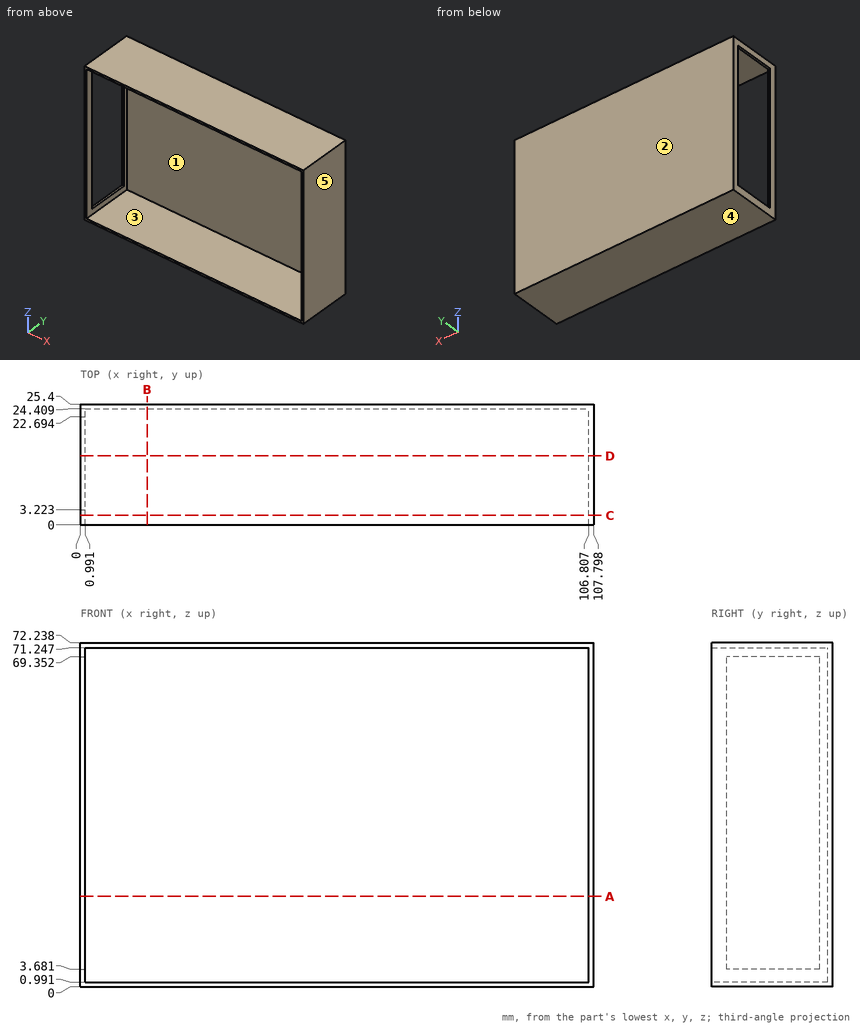
Study the drawing (mm; zero at the part's minimum x, y, z) and answer. A direction names the side the tool comes from. Coordinates: 2 decimals unless noted, no trailing zeros. Loops run counter-clockwise (first coordinate to the right, second up) from the corner with the lowest first, then second, coordinate; pieces in that order, holes last. Notation, with made-up numbers: M 55.5,89 L 63.5,89 A18 ccw 63.5,93 Z; hole C 39.25,75.5 d1. An arc over 180 degrees is marked long. Answer in a Markdown table with one row per item. Add a question column.
1. A tool of negligible diameter and unlimited length cuts with its end or side. For the marked faces 1 and 2, from which of +Z, -Z, +X, -X, +Y, -Y can it reach the whole face along a straight path? Write none if from no direction.
2. The mould has two halves that part along X. Classify the marked faces 3, 4 and 5: pulls with the +X half, pulls with the -X half, needs draft (parallel to the pull), parting line crosses it, or undercut.
3. Find section C-C, the plane y = 2. Write down the section's boundary in (x, z).
4. Find section D-D, the plane y = 14.5. Write down the section's boundary in (x, z).
5. Find section B-B, the plane x = 14. Write down the section's boundary in (y, z), then the cut area to 3 significant figures.
6. Find section A-A, the plane z = 19. Write down the section's boundary in (x, y) (1 decimal), then the cut area to 3 significant figures.
7. Consider L1, parallel to Z at x = 11.5, y = 14.75; L2, parallel to Y at x = 98, z = 60.5; L3, parallel to X at y = 12.25, z = 22. Determine where each line is inside the solid, lowest interval first.
8. Flat-ended cylindrical pins translate along their axes: P1, Ø0.8, axis at x = 0.5, y = 16.5, coming from the -Z side; P2, Ø21, axis at x = 50, z = 34, coming from the -Y side. Find the tip coordinate at first contact, or state that the pin passes through.
Reported:
| question | item | result |
|---|---|---|
| 1 | face 1 | -Y |
| 1 | face 2 | +Z, -Z, +X, -X, +Y |
| 2 | face 3 | undercut |
| 2 | face 4 | needs draft |
| 2 | face 5 | pulls with the +X half |
| 3 | outline | M 0,0 L 107.8,0 L 107.8,72.24 L 0,72.24 Z; hole M 0.99,0.99 L 106.81,0.99 L 106.81,71.25 L 0.99,71.25 Z |
| 4 | outline | M 0,0 L 107.8,0 L 107.8,72.24 L 0,72.24 L 0,69.35 L 0.99,69.35 L 0.99,71.25 L 106.81,71.25 L 106.81,0.99 L 0.99,0.99 L 0.99,3.68 L 0,3.68 Z |
| 5 | outline | M 0,0 L 25.4,0 L 25.4,72.24 L 0,72.24 L 0,71.25 L 24.41,71.25 L 24.41,0.99 L 0,0.99 Z |
| 5 | area | 120 mm^2 |
| 6 | outline | M 0,0 L 1,0 L 1,3.2 L 0,3.2 Z; M 0,22.7 L 1,22.7 L 1,24.4 L 106.8,24.4 L 106.8,0 L 107.8,0 L 107.8,25.4 L 0,25.4 Z |
| 6 | area | 136 mm^2 |
| 7 | L1 | z = 0 to 0.99, 71.25 to 72.24 |
| 7 | L2 | y = 24.41 to 25.4 |
| 7 | L3 | x = 106.81 to 107.8 |
| 8 | P1 | stops at z = 0 |
| 8 | P2 | stops at y = 24.41 |
